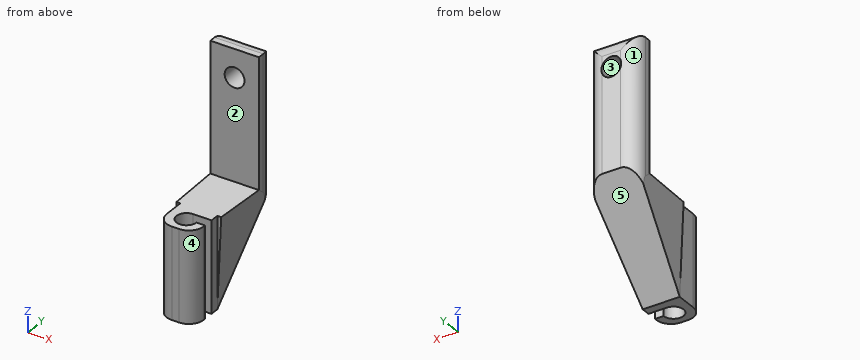
Autodesk Inventor part; units mm, degrees
ref_plane "YZ Plane" through (0, 0, 0) normal (1, 0, 0) x (0, 1, 0)
ref_plane "XZ Plane" through (0, 0, 0) normal (0, 1, 0) x (-1, 0, 0)
ref_plane "XY Plane" through (0, 0, 0) normal (0, 0, 1) x (1, 0, 0)
sketch "Sketch1" plane through (0, 0, 0) normal (0, 1, 0) x (-1, 0, 0)
  circle A0 centre (0, 0) radius 1
  line L0 (0, 1) -> (0, 2.8)
  line L1 (-2.45, 2.8) -> (2.45, 2.8)
  line L2 (2.45, 2.8) -> (2.45, -10.2)
  line L3 (2.45, -10.2) -> (-2.45, -10.2)
  line L4 (-2.45, -10.2) -> (-2.45, 2.8)
  dimension "d0" = 2
  dimension "d1" = 1.8
  dimension "d2" = 4.9
  dimension "d3" = 13
extrude "Extrusion1" add sketch "Sketch1" along normal blind 2.15
sketch "Sketch2" plane through (2.45, 0, 2.8) normal (1, 0, 0) x (0, 0, -1)
  line L0 (0, 0) -> (13, 0)
  line L1 (13, 2.15) -> (13, -5.45)
  line L2 (13, -5.45) -> (22.15, -5.45)
  line L3 (13, 2.15) -> (22.15, -5.45)
  point P0 (2.8, 0)
  dimension "d6" = 7.6
  dimension "d7" = 9.15
extrude "Extrusion2" add sketch "Sketch2" against normal up to surface (4.9 mm away)
sketch "Sketch3" plane through (-2.45, 2.15, -10.2) normal (0, 0.7692539, -0.6389432) x (1, 0, 0)
  line L0 (4.31, 11.8946) -> (0.59, 11.8946)
  line L1 (4.9, 11.8946) -> (0, 11.8946)
  line L2 (4.9, -8.6266) -> (4.9, 1.3737)
  line L3 (4.31, 11.8946) -> (4.9, 1.3737)
  line L4 (0, 1.3737) -> (0, -8.6266)
  line L5 (0.59, 11.8946) -> (0, 1.3737)
  line L6 (4.9, 1.3737) -> (0, 1.3737)
  line L7 (4.9, 1.3737) -> (4.9, 11.8946)
  line L8 (4.9, 11.8946) -> (4.31, 11.8946)
  line L9 (0.59, 11.8946) -> (0, 11.8946)
  line L10 (0, 11.8946) -> (0, 1.3737)
  point P0 (2.45, -6.4727)
  point P1 (2.45, 11.8946)
  point P2 (0.59, 11.8946)
  point P3 (4.31, 11.8946)
  dimension "d10" = 3.72
extrude "Extrusion3" cut sketch "Sketch3" against normal blind 10 contours L1 L7 L3 | L5 L10 L1
sketch "Sketch4" plane through (-2.2547, -5.45, -10.2) normal (0, -1, 0) x (1, 0, 0)
  line L0 (4.1147, -9.15) -> (0.3947, -9.15)
  line L1 (4.7047, 0) -> (-0.1953, 0)
  line L2 (4.1147, -9.15) -> (0.3947, -9.15)
  line L3 (0.3947, -9.15) -> (0.3947, 0)
  line L4 (0.3947, 0) -> (4.1147, 0)
  line L5 (4.1147, 0) -> (4.1147, -9.15)
  point P0 (2.2547, 10.2)
  dimension "d13" = 3.72
extrude "Extrusion4" add sketch "Sketch4" along normal blind 3.56
fillet "Fillet1" radius 1.5 2 edges at (1.86, -9.01, -14.775) (-1.86, -9.01, -14.775)
sketch "Sketch5" plane through (1.86, -5.45, -19.35) normal (0, 0, -1) x (-1, 0, 0)
  circle A0 centre (1.86, -1.875) radius 1
  line L0 (1.86, -0.875) -> (-0.4108, -0.875)
  line L1 (-0.4108, -0.875) -> (-0.4108, -1.875)
  line L2 (-0.4108, -1.875) -> (0.86, -1.875)
  point P0 (1.86, 5.45)
  dimension "d17" = 2
extrude "Extrusion5" cut sketch "Sketch5" against normal through all contours A0
sketch "Sketch6" plane through (1.86, -5.45, -19.35) normal (0, 0, -1) x (-1, 0, 0)
  point P0 (1.86, 5.45)
extrude "Extrusion6" cut sketch "Sketch5" against normal through all contours A0 L2 L1 L0
fillet "Fillet2" radius 1.5 3 edges at (2.45, 2.15, -3.7) (-2.45, 2.15, -3.7) (0, 2.15, 2.8)
Design review of the part built by this model. Coordinates are the model's own, in mm. Face numbers are marked on the shaded views. A direction names the side the tool comes from. Round coordinates to 2 decimals unless told otherwise and drop trailing zeros. Order: outer loops, then holes, each group sorted by start corner. A loop starts at its lowest first (then second) coordinate and runs counter-clockwise, first axis right, second up.
1) Consider section D-D (y = 1.75). State the section outline as (x, z) points, plus the area to 3 significant figures.
The answers:
outline: (-1.97, -10.68) - (1.97, -10.68) - (1.97, 2.32) - (-1.97, 2.32) - close; hole circle Ø2 at (0, 0)
area: 48.1 mm2
2) Consider section A-A (z = 0). State the section outline as (x, y) points, plus the area to 3 significant figures.
The answers:
outline: (-2.45, 0) - (-1, 0) - (-1, 2.15) arc R1.5 ccw to (-2.45, 0.65) - close; (1, 0) - (2.45, 0) - (2.45, 0.65) arc R1.5 ccw to (1, 2.15) - close
area: 5.27 mm2
3) Consider section B-B (x = -0.7). State the section outline as (y, z) points.
The answers:
outline: (-8.97, -19.35) - (-8.04, -19.35) - (-8.04, -10.2) - (-8.97, -10.2) - close; (-6.61, -19.35) - (-5.45, -19.35) - (2.15, -10.2) - (2.15, -0.71) - (0, -0.71) - (0, -10.2) - (-6.61, -10.2) - close; (0, 0.71) - (2.15, 0.71) - (2.15, 1.3) arc R1.5 ccw to (0.65, 2.8) - (0, 2.8) - close
4) Clearance check with flat-ended pins moving along their axes: pin 1 Ø1 at (x, z) = (1, -8.5) entering from -Y; pin 2 Ø1 at (x, y) = (1.5, -3) entering from +Z; pin 3 Ø0.9 at (x, z) = (1, -16.5) entering from -Y. State where each tip first meets the part, or that it passes through.
The answers:
pin 1: stops at y = 0
pin 2: stops at z = -10.2
pin 3: stops at y = -9
5) For L1, parallel to X at y = 1.4, z = 0; L2, parallel to X at y = 0.6, z = 0; L3, parallel to Y at x = -0.05, z = -15.5, list the stretches that pass through material, from the lowest coordinate up.
The answers:
L1: x = -2.25 to -1, 1 to 2.25
L2: x = -2.45 to -1, 1 to 2.45
L3: y = -9.01 to -8.32, -6.33 to -2.25
6) Consider section C-C (z = -2.5). State the section outline as (x, y) points.
The answers:
outline: (-2.45, 0) - (2.45, 0) - (2.45, 0.65) arc R1.5 ccw to (0.95, 2.15) - (-0.95, 2.15) arc R1.5 ccw to (-2.45, 0.65) - close
7) Machinability: for the marked faces 1 and 2, which of the approach directions +Z, -Z, +X, -X, +Y, -Y give a long, thin tool a straight path to every point of the face, cutting with its end or side? Answer none if there is none.
The answers:
face 1: +Z, -Z, -X, +Y
face 2: +Z, +X, -X, -Y
8) Draft analysis for pull direction X (two halves, no side actions). For the marked faces 3, 4 and 5, state which applies: released by +X, released by -X, zero draft, split by the parting line, or undercut.
The answers:
face 3: undercut
face 4: released by +X
face 5: zero draft
